Part model, mm, in its own coordinate system. A direction names the side the tool comes from. Give positions to 0.01 mm unless a question says otherwise; leave off trailing zeros. Write each loop counter-clockwise with the first axis right and the second up, starting at its lowest first coordinate (ties: lowest second). Pieces come first, ordered by that corner, then holes. Notation, with made-up numbers: M -32.75,-37.5 L -19.75,-37.5 A29 cw -19.75,-14.5 Z; hole C 46,-33.5 d1. An arc over 180 degrees is marked long. Use a Markdown table: item, result.
Autodesk Inventor part; units mm, degrees
ref_plane "YZ Plane" through (0, 0, 0) normal (1, 0, 0) x (0, 1, 0)
ref_plane "XZ Plane" through (0, 0, 0) normal (0, 1, 0) x (-1, 0, 0)
ref_plane "XY Plane" through (0, 0, 0) normal (0, 0, 1) x (1, 0, 0)
sketch "Sketch1" plane through (0, 0, 0) normal (1, 0, 0) x (0, 1, 0)
  arc A0 (52.6508, 53.4125) -> (-56.7805, 48.9997) centre (0, 0) ccw
  circle A1 centre (0, 0) radius 7
  arc A2 (-9.1925, -7.7135) -> (9.1925, -7.7135) centre (0, 0) ccw
  line L0 (-9.1925, -7.7135) -> (-56.7805, 48.9997)
  line L1 (0, -37.4043) -> (0, 140.4256)
  line L2 (9.1925, -7.7135) -> (52.6508, 53.4125)
  point P0 (-112.1792, 115.0213)
  point P1 (112.1792, 115.0213)
  dimension "d0" = 150
  dimension "d1" = 14
  dimension "d2" = 5
  dimension "d3" = 40
extrude "Extrusion1" add sketch "Sketch1" along normal blind 10 contours L2 A2 L1 A1 A0 | L1 A1 A2 L0 A0
sketch "Sketch2" plane through (10, 0, 0) normal (1, 0, 0) x (0, 0, -1)
  line L0 (-35, -5.0063) -> (-45, -5.0063)
  line L1 (-45, -5.0063) -> (-45, 4.9937)
  line L2 (-45, 4.9937) -> (-35, 4.9937)
  line L3 (-35, 4.9937) -> (-35, -5.0063)
  point P0 (0, 0)
  dimension "d6" = 10
  dimension "d7" = 10
  dimension "d10" = 35
extrude "Extrusion2" add sketch "Sketch2" along normal blind 50
properties part number "pitch gear v2"
1. Tool access for faces 5 (the cylindrical face through (4.9, -3.9, 74.9)), 6 (the flat face through (4.9, 30.6, 22.4)), 7 (the flat face through (35, 0, 35)), 8 (the flat face through (35, 0, 45)), 9 (the flat face through (35, -5.006, 40)): list every direction of +Z, -Z, +X, -X, +Y, -Y with a clear straight run to the whole face (end or side of a thin tool).
Findings below:
| item | result |
|---|---|
| face 5 | +Z, +X, -X |
| face 6 | -Z, +X, -X, +Y |
| face 7 | -Z, +X, +Y, -Y |
| face 8 | +Z, +X, +Y, -Y |
| face 9 | +Z, -Z, +X, -Y |
2. Drill centre lines: L1, parallel to Z at x = 4.5, y = 0; L2, parallel to X at y = 2, z = 63; L3, parallel to Z at x = 25.5, y = -4. Where is each one in solid material? Low to high.
Findings below:
| item | result |
|---|---|
| L1 | -12 to -7, 7 to 75 |
| L2 | 0 to 10 |
| L3 | 35 to 45 |
3. Two-plate mould, pull along Y, no slides. Class faces 1 (the flat face through (60, 0, 40)), 2 (the cylindrical face through (4.93, 6.466, 2.681)), 3 (the cylindrical face through (5, 0, -12)), 4 (the flat face through (35, 4.994, 40)): released by +Y, released by -Y, zero draft, split by the parting line, or undercut.
Findings below:
| item | result |
|---|---|
| face 1 | zero draft |
| face 2 | undercut |
| face 3 | split by the parting line |
| face 4 | released by +Y |
4. Cut at C-C, the plane x = 43.5. Give the cut face in (y, z), then the cut area to 3 significant figures.
Findings below:
| item | result |
|---|---|
| outline | M -5.01,35 L 4.99,35 L 4.99,45 L -5.01,45 Z |
| area | 100 mm2 |
5. Cut at A-A, the plane y = 0. Give the cut face in (x, z).
Findings below:
| item | result |
|---|---|
| outline | M 0,-12 L 10,-12 L 10,-7 L 0,-7 Z; M 0,7 L 10,7 L 10,35 L 60,35 L 60,45 L 10,45 L 10,75 L 0,75 Z |
6. Cut at B-B, the plane z = 0. Give the cut face in (x, y).
Findings below:
| item | result |
|---|---|
| outline | M 0,-15.66 L 10,-15.66 L 10,-7 L 0,-7 Z; M 0,7 L 10,7 L 10,14.68 L 0,14.68 Z |
7. Drop flat-ended pins along their axis: P1, Ø12, axis at x = 51.5, z = 55.5, coming from the -Y side; P2, Ø5, axis at x = 34, z = 41, coming from the -Y side; P3, Ø8, axis at x = 43, y = -1, coming from the +Z side; P4, Ø10, axis at x = 11, z = 62.5, coming from the +Y side. Give the stop position or say it passes through.
Findings below:
| item | result |
|---|---|
| P1 | through |
| P2 | y = -5.01 |
| P3 | z = 45 |
| P4 | y = 48.03 |
8. Cut at D-D, the plane y = -48. Give the cut face in (x, z).
Findings below:
| item | result |
|---|---|
| outline | M 0,38.54 L 10,38.54 L 10,57.63 L 0,57.63 Z |
